Input: part model. Units: mm. Frame: model coordinates. A direction names the side the tool comes from. Coordinates: 2 decimals unless noted, no trailing zeros. Order: outer loops, then holes, each group sorted by start corner. A loop starts at its lowest first (then second) coordinate and runs counter-clockwise, first axis right, second up.
from build123d import *

# Parameters (mm, degrees)
SKETCH1_R           = 3.4036
BOSS_EXTRUDE1_DEPTH = 127


with BuildPart() as part:
    # Sketch1 → Boss-Extrude1 (new, symmetric)
    with BuildSketch(Plane(origin=(0, 0, 0), x_dir=(1, 0, 0), z_dir=(0, 1, 0))):
        with BuildLine():
            Line((-20, 16.952), (-20, 4.7625))
            ThreePointArc((-20, 4.7625), (-19.776815367, 4.223684633), (-19.238, 4.0005))
            Line((-19.238, 4.0005), (-16.2662, 4.0005))
            ThreePointArc((-16.2662, 4.0005), (-15.727384633, 4.223684633), (-15.5042, 4.7625))
            Line((-15.5042, 4.7625), (-15.5042, 10.2235))
            ThreePointArc((-15.5042, 10.2235), (-15.033804775, 10.927496204), (-14.203384633, 10.762315367))
            Line((-14.203384633, 10.762315367), (-8.635059555, 5.19399029))
            ThreePointArc((-8.635059555, 5.19399029), (-7.985348265, 4.221628629), (-7.7572, 3.074649845))
            Line((-7.7572, 3.074649845), (-7.7572, -3.074649845))
            ThreePointArc((-7.7572, -3.074649845), (-7.985348265, -4.221628629), (-8.635059555, -5.19399029))
            Line((-8.635059555, -5.19399029), (-14.203384633, -10.762315367))
            ThreePointArc((-14.203384633, -10.762315367), (-15.033804775, -10.927496204), (-15.5042, -10.2235))
            Line((-15.5042, -10.2235), (-15.5042, -4.7625))
            ThreePointArc((-15.5042, -4.7625), (-15.727384633, -4.223684633), (-16.2662, -4.0005))
            Line((-16.2662, -4.0005), (-19.238, -4.0005))
            ThreePointArc((-19.238, -4.0005), (-19.776815367, -4.223684633), (-20, -4.7625))
            Line((-20, -4.7625), (-20, -16.952))
            ThreePointArc((-20, -16.952), (-19.107261469, -19.107261469), (-16.952, -20))
            Line((-16.952, -20), (-4.7625, -20))
            ThreePointArc((-4.7625, -20), (-4.223684633, -19.776815367), (-4.0005, -19.238))
            Line((-4.0005, -19.238), (-4.0005, -16.2662))
            ThreePointArc((-4.0005, -16.2662), (-4.223684633, -15.727384633), (-4.7625, -15.5042))
            Line((-4.7625, -15.5042), (-10.2235, -15.5042))
            ThreePointArc((-10.2235, -15.5042), (-10.927496204, -15.033804775), (-10.762315367, -14.203384633))
            Line((-10.762315367, -14.203384633), (-5.19399029, -8.635059555))
            ThreePointArc((-5.19399029, -8.635059555), (-4.221628629, -7.985348265), (-3.074649845, -7.7572))
            Line((-3.074649845, -7.7572), (3.074649845, -7.7572))
            ThreePointArc((3.074649845, -7.7572), (4.221628629, -7.985348265), (5.19399029, -8.635059555))
            Line((5.19399029, -8.635059555), (10.762315367, -14.203384633))
            ThreePointArc((10.762315367, -14.203384633), (10.927496204, -15.033804775), (10.2235, -15.5042))
            Line((10.2235, -15.5042), (4.7625, -15.5042))
            ThreePointArc((4.7625, -15.5042), (4.223684633, -15.727384633), (4.0005, -16.2662))
            Line((4.0005, -16.2662), (4.0005, -19.238))
            ThreePointArc((4.0005, -19.238), (4.223684633, -19.776815367), (4.7625, -20))
            Line((4.7625, -20), (16.952, -20))
            ThreePointArc((16.952, -20), (19.107261469, -19.107261469), (20, -16.952))
            Line((20, -16.952), (20, -4.7625))
            ThreePointArc((20, -4.7625), (19.776815367, -4.223684633), (19.238, -4.0005))
            Line((19.238, -4.0005), (16.2662, -4.0005))
            ThreePointArc((16.2662, -4.0005), (15.727384633, -4.223684633), (15.5042, -4.7625))
            Line((15.5042, -4.7625), (15.5042, -10.2235))
            ThreePointArc((15.5042, -10.2235), (15.033804775, -10.927496204), (14.203384633, -10.762315367))
            Line((14.203384633, -10.762315367), (8.635059555, -5.19399029))
            ThreePointArc((8.635059555, -5.19399029), (7.985348265, -4.221628629), (7.7572, -3.074649845))
            Line((7.7572, -3.074649845), (7.7572, 3.074649845))
            ThreePointArc((7.7572, 3.074649845), (7.985348265, 4.221628629), (8.635059555, 5.19399029))
            Line((8.635059555, 5.19399029), (14.203384633, 10.762315367))
            ThreePointArc((14.203384633, 10.762315367), (15.033804775, 10.927496204), (15.5042, 10.2235))
            Line((15.5042, 10.2235), (15.5042, 4.7625))
            ThreePointArc((15.5042, 4.7625), (15.727384633, 4.223684633), (16.2662, 4.0005))
            Line((16.2662, 4.0005), (19.238, 4.0005))
            ThreePointArc((19.238, 4.0005), (19.776815367, 4.223684633), (20, 4.7625))
            Line((20, 4.7625), (20, 16.952))
            ThreePointArc((20, 16.952), (19.107261469, 19.107261469), (16.952, 20))
            Line((16.952, 20), (4.7625, 20))
            ThreePointArc((4.7625, 20), (4.223684633, 19.776815367), (4.0005, 19.238))
            Line((4.0005, 19.238), (4.0005, 16.2662))
            ThreePointArc((4.0005, 16.2662), (4.223684633, 15.727384633), (4.7625, 15.5042))
            Line((4.7625, 15.5042), (10.2235, 15.5042))
            ThreePointArc((10.2235, 15.5042), (10.927496204, 15.033804775), (10.762315367, 14.203384633))
            Line((10.762315367, 14.203384633), (5.19399029, 8.635059555))
            ThreePointArc((5.19399029, 8.635059555), (4.221628629, 7.985348265), (3.074649845, 7.7572))
            Line((3.074649845, 7.7572), (-3.074649845, 7.7572))
            ThreePointArc((-3.074649845, 7.7572), (-4.221628629, 7.985348265), (-5.19399029, 8.635059555))
            Line((-5.19399029, 8.635059555), (-10.762315367, 14.203384633))
            ThreePointArc((-10.762315367, 14.203384633), (-10.927496204, 15.033804775), (-10.2235, 15.5042))
            Line((-10.2235, 15.5042), (-4.7625, 15.5042))
            ThreePointArc((-4.7625, 15.5042), (-4.223684633, 15.727384633), (-4.0005, 16.2662))
            Line((-4.0005, 16.2662), (-4.0005, 19.238))
            ThreePointArc((-4.0005, 19.238), (-4.223684633, 19.776815367), (-4.7625, 20))
            Line((-4.7625, 20), (-16.952, 20))
            ThreePointArc((-16.952, 20), (-19.107261469, 19.107261469), (-20, 16.952))
        make_face()
        with Locations(Location((0, 0, 0), (0, 0, 270))):
            Circle(SKETCH1_R, mode=Mode.SUBTRACT)
    extrude(amount=BOSS_EXTRUDE1_DEPTH, both=True)


solid = part.part
Item 1: Draft query along Z for faces 4 (the face through (0, 2, -7.757)), 5 (the face through (4, -127, 0)), 6 (the face through (-11.38, 1.78, 7.94)). Return one class per face: pulls with the +Z half, pulls with the -Z half, needs draft (parallel to the pull), parting line crosses it, or undercut.
Response values:
face 4: pulls with the -Z half
face 5: needs draft
face 6: undercut
Item 2: Ray query, probe 1 along X at (y, z) = (23, 0); probe 2 along Z at (x, y) = (-14.5, -32); probe 3 along Z at (x, y) = (-7, 62.5). Return the intervals inside material, ascending.
Response values:
probe 1: x = -7.76 to -3.4, 3.4 to 7.76
probe 2: z = -20 to -10.95, 10.95 to 20
probe 3: z = -20 to -15.5, -10.44 to 10.44, 15.5 to 20
Item 3: Cut plane B-B on z = 0. Return loops of the section in (x, y).
Response values:
outline: (-7.76, -127) - (-3.4, -127) - (-3.4, 127) - (-7.76, 127) - close; (3.4, -127) - (7.76, -127) - (7.76, 127) - (3.4, 127) - close
Item 4: Access query for faces 1 (the face through (11, 2, 20)), 2 (the face through (7.94, 1.78, 11.38)), 3 (the face through (-7.757, 2, 0)). Directions: +Z, -Z, +X, -X, +Y, -Y. A direction counts if a zero-diameter tool reaches every point of the face in a straight line with its end or side. Return the directions, or none.
Response values:
face 1: +Z, +X, -X, +Y, -Y
face 2: +Y, -Y
face 3: -X, +Y, -Y
Item 5: Pin query (flat end, axial travel): pin 1 Ø2 at (x, y) = (-2, -33.5) entering from +Z; pin 2 Ø7 at (x, y) = (-1, 33.5) entering from -Z; pin 3 Ø5 at (y, z) = (-45, 0.5) entering from -X. Return the tip coordinate at first contact, or that it passes through.
Response values:
pin 1: stops at z = 7.76
pin 2: stops at z = -19.95
pin 3: stops at x = -7.76
Item 6: Cut plane A-A on x = 0. Return loops of the section in (y, z), then the cut area to 3 significant figures.
Response values:
outline: (-127, -7.76) - (127, -7.76) - (127, -3.4) - (-127, -3.4) - close; (-127, 3.4) - (127, 3.4) - (127, 7.76) - (-127, 7.76) - close
area: 2,210 mm2
